```python
from build123d import *

# Parameters (mm, degrees)
SKETCH1_R           = 2.2225
BOSS_EXTRUDE1_DEPTH = 6.35
FILLET1_R           = 2.54


with BuildPart() as part:
    # Sketch1 → Boss-Extrude1 (new body)
    with BuildSketch(Plane(origin=(0, 0, 0), x_dir=(1, 0, 0), z_dir=(0, 1, 0))):
        Polygon((-38.1, 0), (-20.32, 0), (-20.32, -12.7), (20.32, -12.7), (20.32, 0), (38.1, 0), (38.1, -25.4), (25.4, -25.4), (25.4, -38.1), (15.24, -38.1), (15.24, -25.4), (-15.24, -25.4), (-15.24, -38.1), (-25.4, -38.1), (-25.4, -25.4), (-38.1, -25.4), align=None)
        with Locations(Location((-28.702, -12.7, 0), (0, 0, 270))):
            Circle(SKETCH1_R, mode=Mode.SUBTRACT)
        with Locations(Location((28.702, -12.7, 0), (0, 0, 270))):
            Circle(SKETCH1_R, mode=Mode.SUBTRACT)
        with BuildLine():
            Line((-18.0975, -27.94), (-18.0975, -34.29))
            ThreePointArc((-18.0975, -34.29), (-20.32, -36.5125), (-22.5425, -34.29))
            Line((-22.5425, -34.29), (-22.5425, -27.94))
            ThreePointArc((-22.5425, -27.94), (-20.32, -25.7175), (-18.0975, -27.94))
        make_face(mode=Mode.SUBTRACT)
        with BuildLine():
            Line((18.0975, -27.94), (18.0975, -34.29))
            ThreePointArc((18.0975, -34.29), (20.32, -36.5125), (22.5425, -34.29))
            Line((22.5425, -34.29), (22.5425, -27.94))
            ThreePointArc((22.5425, -27.94), (20.32, -25.7175), (18.0975, -27.94))
        make_face(mode=Mode.SUBTRACT)
    extrude(amount=BOSS_EXTRUDE1_DEPTH)

    # Fillet1
    fillet1_edges = [part.edges().sort_by_distance(p)[0] for p in [
        (38.1, 3.175, 0),
        (38.1, 3.175, 25.4),
        (25.4, 3.175, 25.4),
        (25.4, 3.175, 38.1),
        (15.24, 3.175, 38.1),
        (15.24, 3.175, 25.4),
        (-15.24, 3.175, 25.4),
        (-15.24, 3.175, 38.1),
        (-25.4, 3.175, 38.1),
        (-25.4, 3.175, 25.4),
        (-38.1, 3.175, 25.4),
        (-38.1, 3.175, 0),
        (-20.32, 3.175, 0),
        (-20.32, 3.175, 12.7),
        (20.32, 3.175, 12.7),
        (20.32, 3.175, 0),
    ]]
    fillet(fillet1_edges, radius=FILLET1_R)


solid = part.part
```
Work out the finished part from the listing and answer in its coordinate system (mm). A direction names the side the tool comes from. Give positions to 0.01 mm unless a question says otherwise; leave off trailing zeros. Write each loop counter-clockwise with the first axis right and the second up, starting at its lowest first coordinate (ties: lowest second). Pieces come first, ordered by that corner, then holes.
(1) The part is cut by section A-A on z = 4. Write down the section's boundary in (x, y), plus the area to 3 significant figures.
Final values:
outline: (-38.1, 0) - (-20.32, 0) - (-20.32, 6.35) - (-38.1, 6.35) - close; (20.32, 0) - (38.1, 0) - (38.1, 6.35) - (20.32, 6.35) - close
area: 226 mm2
(2) Flat-ended cylindrical pins translate along their axes: pin 1 Ø1.9 at (y, z) = (3.5, 30) entering from +X; pin 2 Ø3 at (x, y) = (8, 3.5) entering from +Z; pin 3 Ø1 at (x, y) = (8, 2) entering from -Z. Find the tip coordinate at first contact, or state that the pin passes through.
Final values:
pin 1: stops at x = 25.4
pin 2: stops at z = 25.4
pin 3: stops at z = 12.7
(3) The part is cut by section B-B on z = 31. Write down the section's boundary in (x, y).
Final values:
outline: (-25.4, 0) - (-22.54, 0) - (-22.54, 6.35) - (-25.4, 6.35) - close; (-18.1, 0) - (-15.24, 0) - (-15.24, 6.35) - (-18.1, 6.35) - close; (15.24, 0) - (18.1, 0) - (18.1, 6.35) - (15.24, 6.35) - close; (22.54, 0) - (25.4, 0) - (25.4, 6.35) - (22.54, 6.35) - close
(4) The mould has two halves that part along Z. Classify faces 5 (the cylindrical face through (37.376, 3.219, 24.636)), 6 (the cylindrical face through (-26.5, 3.1, 12.4)), 7 (the flat face through (38.1, 3, 13)), 8 (the cylindrical face through (21.044, 3.219, 0.764)): pulls with the +Z half, pulls with the -Z half, needs draft (parallel to the pull), parting line crosses it, or undercut.
Final values:
face 5: pulls with the +Z half
face 6: undercut
face 7: needs draft
face 8: pulls with the -Z half
(5) The part is cut by section C-C on y = 1.75. Count the separate pieces of the cut face and the enclosed holes in it, plus the area to 3 significant figures.
Final values:
separate pieces: 1
enclosed holes: 4
area: 1,550 mm2
(6) The part is cut by section D-D on x = -17. Write down the section's boundary in (y, z).
Final values:
outline: (0, 12.7) - (6.35, 12.7) - (6.35, 37.98) - (0, 37.98) - close
(7) Straight lines are drawn through the part: line 1 (X direction, y = 5.25, z = 32); line 2 (X direction, y = 3.5, z = 2.5); line 3 (X direction, y = 5, z = 27). For each, find the intervals that lie inside material, in ascending order.
Final values:
line 1: x = -25.4 to -22.54, -18.1 to -15.24, 15.24 to 18.1, 22.54 to 25.4
line 2: x = -38.1 to -20.32, 20.32 to 38.1
line 3: x = -25.58 to -22.33, -18.31 to -15.06, 15.06 to 18.31, 22.33 to 25.58
(8) Which of the six approach directions +Z, -Z, +X, -X, +Y, -Y give full straight-line access (tool end or side, diameter ignored) to faces 1 (the flat face through (-25.4, 3, 32)), 2 (the flat face through (-15.24, 3, 32)), 3 (the flat face through (22.542, 3, 31)), 4 (the flat face through (-20, 3, 38.1))?
Final values:
face 1: +Z, -X, +Y, -Y
face 2: +Z, +Y, -Y
face 3: +Y, -Y
face 4: +Z, +X, -X, +Y, -Y
